Check sheet for the modelled part. Datum: model origin and axes. Units: mm. A direction names the side the tool comes from. Give positions to 0.01 mm unless a question says otherwise; leave off trailing zeros. Order: outer loops, then holes, each group sorted by start corner. A loop starts at its lowest first (then second) coordinate and runs counter-clockwise, first axis right, second up.
```python
from build123d import *

# Parameters (mm, degrees)
CROQUIS1_R              = 50
SALIENTE_EXTRUIR1_DEPTH = 30
CROQUIS2_R              = 40.25
CORTAR_EXTRUIR1_DEPTH   = 10.5
CROQUIS3_R              = 21.5
SALIENTE_EXTRUIR2_DEPTH = 12.9
CORTAR_EXTRUIR2_DEPTH   = 12.9
CROQUIS7_W              = 44
CROQUIS7_H              = 8
SALIENTE_EXTRUIR3_DEPTH = 82.4
REDONDEO1_R             = 5
CORTAR_EXTRUIR3_REACH   = 146.079
CROQUIS8_R              = 1.1
CROQUIS9_R              = 1.5
CORTAR_EXTRUIR4_DEPTH   = 7
CROQUIS11_R             = 1.25
CORTAR_EXTRUIR5_DEPTH   = 15
SALIENTE_EXTRUIR4_START = 10.5
CROQUIS12_R             = 40.25
CROQUIS12_R_2           = 37.68
SALIENTE_EXTRUIR4_DEPTH = 10.5
CORTAR_EXTRUIR6_REACH   = 126.031
CROQUIS13_R             = 5
CROQUIS14_W             = 27
CROQUIS14_H             = 10
CORTAR_EXTRUIR7_DEPTH   = 5
CORTAR_EXTRUIR8_START   = -2.5
CROQUIS15_R             = 35
CROQUIS15_R_2           = 21.5
CORTAR_EXTRUIR8_DEPTH   = 2.5


with BuildPart() as part:
    # Croquis1 → Saliente-Extruir1 (new body)
    with BuildSketch(Plane.XY):
        Circle(CROQUIS1_R)
    extrude(amount=SALIENTE_EXTRUIR1_DEPTH)

    # Croquis2 → Cortar-Extruir1 (cut)
    with BuildSketch(Plane(origin=(0, 0, 0), x_dir=(-1, 0, 0), z_dir=(0, 0, -1))):
        Circle(CROQUIS2_R)
    extrude(amount=-CORTAR_EXTRUIR1_DEPTH, mode=Mode.SUBTRACT)

    # Croquis3 → Saliente-Extruir2 (add)
    with BuildSketch(Plane(origin=(0, 0, 10.5), x_dir=(-1, 0, 0), z_dir=(0, 0, -1))):
        with Locations(Location((0, 0, 0), (0, 0, 180))):
            Circle(CROQUIS3_R)
    extrude(amount=SALIENTE_EXTRUIR2_DEPTH)

    # Croquis4 → Cortar-Extruir2 (cut)
    with BuildSketch(Plane(origin=(0, 0, -2.4), x_dir=(-1, 0, 0), z_dir=(0, 0, -1))):
        with BuildLine():
            ThreePointArc((-0.668583659, -6.566048727), (0.596468383, -7.752086846), (1.665189454, -6.386481354))
            ThreePointArc((1.665189454, -6.386481354), (2.986052332, -5.885872193), (4.170137542, -5.11565762))
            ThreePointArc((4.170137542, -5.11565762), (5.903320016, -5.059786339), (5.693391028, -3.338457518))
            ThreePointArc((5.693391028, -3.338457518), (6.273397994, -2.050482288), (6.566048727, -0.668583659))
            ThreePointArc((6.566048727, -0.668583659), (7.752086846, 0.596468383), (6.386481354, 1.665189454))
            ThreePointArc((6.386481354, 1.665189454), (5.885872193, 2.986052332), (5.11565762, 4.170137542))
            ThreePointArc((5.11565762, 4.170137542), (5.059786339, 5.903320016), (3.338457518, 5.693391028))
            ThreePointArc((3.338457518, 5.693391028), (2.050482288, 6.273397994), (0.668583659, 6.566048727))
            ThreePointArc((0.668583659, 6.566048727), (-0.596468383, 7.752086846), (-1.665189454, 6.386481354))
            ThreePointArc((-1.665189454, 6.386481354), (-2.986052332, 5.885872193), (-4.170137542, 5.11565762))
            ThreePointArc((-4.170137542, 5.11565762), (-5.903320016, 5.059786339), (-5.693391028, 3.338457518))
            ThreePointArc((-5.693391028, 3.338457518), (-6.273397994, 2.050482288), (-6.566048727, 0.668583659))
            ThreePointArc((-6.566048727, 0.668583659), (-7.752086846, -0.596468383), (-6.386481354, -1.665189454))
            ThreePointArc((-6.386481354, -1.665189454), (-5.885872193, -2.986052332), (-5.11565762, -4.170137542))
            ThreePointArc((-5.11565762, -4.170137542), (-5.059786339, -5.903320016), (-3.338457518, -5.693391028))
            ThreePointArc((-3.338457518, -5.693391028), (-2.050482288, -6.273397994), (-0.668583659, -6.566048727))
        make_face()
    extrude(amount=-CORTAR_EXTRUIR2_DEPTH, mode=Mode.SUBTRACT)

    # Croquis7 → Saliente-Extruir3 (add)
    with BuildSketch(Plane.XY.offset(30)):
        with Locations((0, -21)):
            Rectangle(CROQUIS7_W, CROQUIS7_H)
        with Locations((0, 21)):
            Rectangle(CROQUIS7_W, CROQUIS7_H)
    extrude(amount=SALIENTE_EXTRUIR3_DEPTH)

    # Redondeo1
    redondeo1_edges = [part.edges().sort_by_distance(p)[0] for p in [
        (22, -21, 30),
        (-22, -21, 30),
        (0, -25, 30),
        (22, 21, 30),
        (0, 25, 30),
        (-22, 21, 30),
    ]]
    fillet(redondeo1_edges, radius=REDONDEO1_R)

    # Cortar-Extruir3: up to this face of the body (flat: up to its plane)
    cortar_extruir3_end = Plane(part.part.faces().sort_by_distance((0, 25, 73.7))[0])
    # Croquis8 → Cortar-Extruir3 (cut, up to the picked face)
    with BuildSketch(Plane.XZ.offset(25), mode=Mode.PRIVATE) as cortar_extruir3_sk1:
        with Locations(Location((-8, 36.75, 0), (0, 0, 270))):
            Circle(CROQUIS8_R)
    cortar_extruir3_tool1 = split(extrude(cortar_extruir3_sk1.sketch, amount=-CORTAR_EXTRUIR3_REACH, mode=Mode.PRIVATE), bisect_by=cortar_extruir3_end, keep=Keep.BOTH, mode=Mode.PRIVATE)
    # Croquis8 → Cortar-Extruir3 (cut, up to the picked face)
    with BuildSketch(Plane.XZ.offset(25), mode=Mode.PRIVATE) as cortar_extruir3_sk2:
        with Locations(Location((8, 36.75, 0), (0, 0, 270))):
            Circle(CROQUIS8_R)
    cortar_extruir3_tool2 = split(extrude(cortar_extruir3_sk2.sketch, amount=-CORTAR_EXTRUIR3_REACH, mode=Mode.PRIVATE), bisect_by=cortar_extruir3_end, keep=Keep.BOTH, mode=Mode.PRIVATE)
    # Croquis8 → Cortar-Extruir3 (cut, up to the picked face)
    with BuildSketch(Plane.XZ.offset(25), mode=Mode.PRIVATE) as cortar_extruir3_sk3:
        with Locations(Location((-8, 68.75, 0), (0, 0, 270))):
            Circle(CROQUIS8_R)
    cortar_extruir3_tool3 = split(extrude(cortar_extruir3_sk3.sketch, amount=-CORTAR_EXTRUIR3_REACH, mode=Mode.PRIVATE), bisect_by=cortar_extruir3_end, keep=Keep.BOTH, mode=Mode.PRIVATE)
    # Croquis8 → Cortar-Extruir3 (cut, up to the picked face)
    with BuildSketch(Plane.XZ.offset(25), mode=Mode.PRIVATE) as cortar_extruir3_sk4:
        with Locations(Location((8, 68.75, 0), (0, 0, 270))):
            Circle(CROQUIS8_R)
    cortar_extruir3_tool4 = split(extrude(cortar_extruir3_sk4.sketch, amount=-CORTAR_EXTRUIR3_REACH, mode=Mode.PRIVATE), bisect_by=cortar_extruir3_end, keep=Keep.BOTH, mode=Mode.PRIVATE)
    add(cortar_extruir3_tool1.solids().sort_by(Axis((-8, -25, 36.75), (0, 1, 0)))[0], mode=Mode.SUBTRACT)
    add(cortar_extruir3_tool2.solids().sort_by(Axis((8, -25, 36.75), (0, 1, 0)))[0], mode=Mode.SUBTRACT)
    add(cortar_extruir3_tool3.solids().sort_by(Axis((-8, -25, 68.75), (0, 1, 0)))[0], mode=Mode.SUBTRACT)
    add(cortar_extruir3_tool4.solids().sort_by(Axis((8, -25, 68.75), (0, 1, 0)))[0], mode=Mode.SUBTRACT)

    # Croquis9 → Cortar-Extruir4 (cut)
    with BuildSketch(Plane.XY.offset(30)):
        with Locations((-42, 0)):
            Circle(CROQUIS9_R)
        with Locations((-21, 36.373066959)):
            Circle(CROQUIS9_R)
        with Locations((21, 36.373066959)):
            Circle(CROQUIS9_R)
        with Locations((42, 0)):
            Circle(CROQUIS9_R)
        with Locations((21, -36.373066959)):
            Circle(CROQUIS9_R)
        with Locations((-21, -36.373066959)):
            Circle(CROQUIS9_R)
    extrude(amount=-CORTAR_EXTRUIR4_DEPTH, mode=Mode.SUBTRACT)

    # Croquis11 → Cortar-Extruir5 (cut)
    with BuildSketch(Plane.XY.offset(112.4)):
        with Locations((-18, -21)):
            Circle(CROQUIS11_R)
        with Locations((18, -21)):
            Circle(CROQUIS11_R)
        with Locations((-18, 21)):
            Circle(CROQUIS11_R)
        with Locations((18, 21)):
            Circle(CROQUIS11_R)
    extrude(amount=-CORTAR_EXTRUIR5_DEPTH, mode=Mode.SUBTRACT)

    # Croquis12 → Saliente-Extruir4 (add)
    with BuildSketch(Plane(origin=(0, 0, 10.5), x_dir=(-1, 0, 0), z_dir=(0, 0, -1)).offset(SALIENTE_EXTRUIR4_START)):
        Circle(CROQUIS12_R)
        with Locations(Location((0, 0, 0), (0, 0, 180))):
            Circle(CROQUIS12_R_2, mode=Mode.SUBTRACT)
    extrude(amount=-SALIENTE_EXTRUIR4_DEPTH)

    # Croquis13 → Cortar-Extruir6 (cut, up to next)
    with BuildSketch(Plane(origin=(0, 0, 10.5), x_dir=(-1, 0, 0), z_dir=(0, 0, -1)), mode=Mode.PRIVATE) as cortar_extruir6_sk1:
        Circle(CROQUIS13_R)
    cortar_extruir6_tool1 = extrude(cortar_extruir6_sk1.sketch, amount=-CORTAR_EXTRUIR6_REACH, mode=Mode.PRIVATE) & part.part
    add(cortar_extruir6_tool1.solids().sort_by_distance((0, 0, 10.5))[0], mode=Mode.SUBTRACT)

    # Croquis14 → Cortar-Extruir7 (cut)
    with BuildSketch(Plane.XY.offset(30)):
        with Locations((-13.5, 0)):
            Rectangle(CROQUIS14_W, CROQUIS14_H)
    extrude(amount=-CORTAR_EXTRUIR7_DEPTH, mode=Mode.SUBTRACT)

    # Croquis15 → Cortar-Extruir8 (cut)
    with BuildSketch(Plane(origin=(0, 0, 10.5), x_dir=(-1, 0, 0), z_dir=(0, 0, -1)).offset(CORTAR_EXTRUIR8_START)):
        Circle(CROQUIS15_R)
        with Locations(Location((0, 0, 0), (0, 0, 180))):
            Circle(CROQUIS15_R_2, mode=Mode.SUBTRACT)
    extrude(amount=CORTAR_EXTRUIR8_DEPTH, mode=Mode.SUBTRACT)


solid = part.part
```
(1) Go/stop test with flat-tipped pins: P1, Ø5, axis at x = -14.5, y = -1.5, coming from the +Z side; P2, Ø4, axis at x = -20.5, y = 35, coming from the +Z side; P3, Ø8, axis at x = 22, z = 28, coming from the -Y side. Record where each tip stops, or that it passes through.
(2) Thickness scan on L1, parallel to Y at x = -12.5, z = 82; L2, parallel to Y at x = 0, z = 24.5; L3, parallel to Y at x = -21, z = 26. Record the ranges inside material, lowest first.
(3) Sectioned sample at B-B (x = -42). Enter the section's corners in (y, z), plus the area to 3 significant figures.
(4) Release check for a two-part mould opening along Y. For faces 6 (the face through (47.69, 15.02, 14.79)), 7 (the face through (-24, 22, 31)), 8 (the face through (10, 1, 30)) record: released by +Y, released by -Y, zero draft, split by the parting line, or undercut.
(5) Tool access check on faces 1 (the face through (-22, -21, 73)), 2 (the face through (22, -21, 73)), 3 (the face through (0, 17, 71)), 4 (the face through (-21, 36, 23)), 5 (the face through (-2.799, -21.317, 5.408)). Record the directions out of +Z, -Z, +X, -X, +Y, -Y that give a thin tool (end or side, any length) a straight path to the whole face; none if there is none.
(6) Sectioned sample at D-D (y = -32). Enter the section's corners in (x, z).
(7) Sectioned sample at A-A (z = 31.5). Enter the section's corners in (x, y), plus the area to 3 significant figures.
(8) Sectioned sample at C-C (z = 89.5). Enter the section's corners in (x, y).
Values follow:
1. P1: stops at z = 25
1. P2: stops at z = 30
1. P3: stops at y = -46.65
2. L1: y = -25 to -17, 17 to 25
2. L2: y = -50 to -5, 5 to 50
2. L3: y = -45.38 to -37.87, -34.87 to -5, 5 to 34.87, 37.87 to 45.38
3. outline: (-27.13, 0) - (27.13, 0) - (27.13, 30) - (1.5, 30) - (1.5, 23) - (-1.5, 23) - (-1.5, 30) - (-27.13, 30) - close
3. area: 1,610 mm2
4. face 6: split by the parting line
4. face 7: zero draft
4. face 8: undercut
5. face 1: +Z, -X, +Y, -Y
5. face 2: +Z, +X, +Y, -Y
5. face 3: +Z, +X, -X
5. face 4: +Z
5. face 5: -Z
6. outline: (-38.42, 0) - (-19.89, 0) - (-19.89, 10.5) - (-14.18, 10.5) - (-14.18, 13) - (14.18, 13) - (14.18, 10.5) - (19.89, 10.5) - (19.89, 0) - (38.42, 0) - (38.42, 30) - (-38.42, 30) - close
7. outline: (-23.43, -26.43) - (23.43, -26.43) - (23.43, -17) - (-23.43, -17) - close; (-23.43, 17) - (23.43, 17) - (23.43, 26.43) - (-23.43, 26.43) - close
7. area: 884 mm2
8. outline: (-22, -25) - (22, -25) - (22, -17) - (-22, -17) - close; (-22, 17) - (22, 17) - (22, 25) - (-22, 25) - close
